Answer from the drawing. Dimensions are ordinates in mm from the lowest x, y and z of the part. A direction names the side the tool comes from. Give positions to 0.01 mm unless a question says otherwise; leave off trailing zeros. Write each loop counter-clockwise with the first axis right and the second up, starting at its lowest first coordinate (ties: lowest second). Pieces come first, ordered by that corner, then holes. Notation, with made-up numbers: M 15,21.5 L 27,21.5 A12 cw 27,38.5 Z; hole C -8,39 d3. An arc over 180 degrees is marked long. Put each result on its own line as item: value.
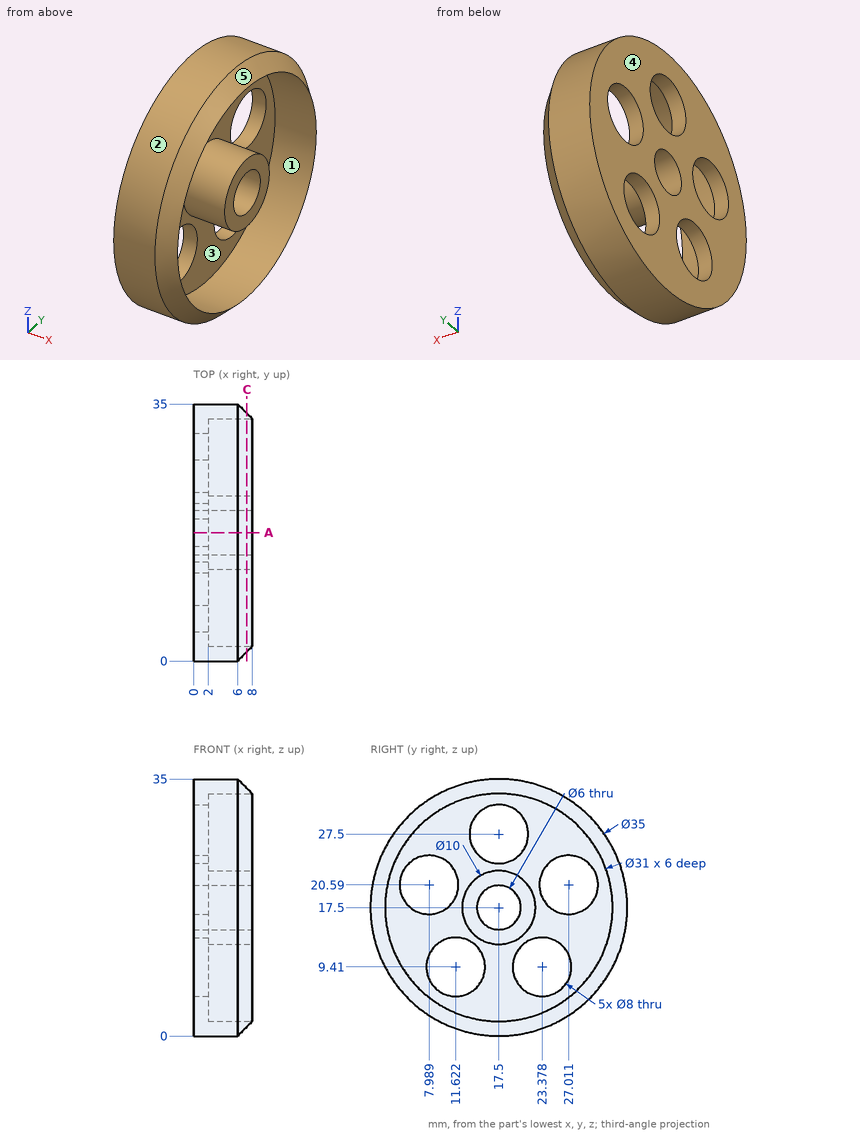
(1) Section A-A on y = 17.5 is taken. Give the number of separate pieces and of enclosed holes in the cut face.
Result:
separate pieces: 3
enclosed holes: 0
(2) Which of the six approach directions +Z, -Z, +X, -X, +Y, -Y give full straight-line access (tool end or side, diameter ignored) to the marked faces 1 and 2?
Result:
face 1: +X
face 2: +X, -X
(3) Given pin 1 Ø10 at (y, z) = (19, 25) entering from -X; pin 2 Ø1.5 at (x, y) = (2, 8) entering from +Z (1 decimal), each flat-ended and moving along its own axis, determine where each tip first touches the part or whether it passes through.
Result:
pin 1: stops at x = 0
pin 2: stops at z = 32.7
(4) For a pull along Z with two mould halves and no side action, classify the marked faces 3, 4 and 5 as +Z half, -Z half, draft (parallel to the pull), parting line (faces both ways), or undercut.
Result:
face 3: undercut
face 4: draft
face 5: parting line
(5) Straight lines are drawn through the part: line 1 along Z through (x, y) = (0.8, 17.5); line 2 along Y through (x, z) = (7.75, 13) (1 decimal); line 3 along Z through (x, y) = (1.5, 25.5) (1 decimal). For each, find the intervals that lie inside material, in ascending order. Write a range as from..to.
Result:
line 1: z = 0..14.5, 20.5..23.5, 31.5..35
line 2: y = 2.4..2.7, 15.3..19.7, 32.3..32.6
line 3: z = 1.9..6, 12.8..16.9, 24.3..33.1
(6) Section C-C on x = 7.25 is taken. Determine the outline of the cut face in (y, z), and give its area (3 significant figures).
Result:
outline: C 17.5,17.5 d32.5; C 17.5,17.5 d10; hole C 17.5,17.5 d31; hole C 17.5,17.5 d6
area: 125 mm²
